```python
from build123d import *

# Parameters (mm, degrees)
SKETCH1_W                      = 40
SKETCH1_H                      = 45.36
BOSS_EXTRUDE1_DEPTH            = 14
SKETCH2_W                      = 29.2
SKETCH2_H                      = 38.5
CUT_EXTRUDE1_DEPTH             = 6.2
M2_5_CLEARANCE_HOLE1_OUTLINE_R = 1.45
M2_5_CLEARANCE_HOLE1_DEPTH     = 14
F_16_0MM_DOWEL_HOLE1_D         = 16
SKETCH11_R                     = 16
CUT_EXTRUDE2_DEPTH             = 63.076804041
CHAMFER1_SIZE                  = 6
FILLET1_R                      = 2


# Read off the part's stored shape, not the designer's step: M2.5 Clearance Hole1
with BuildPart() as part:
    # Sketch1 → Boss-Extrude1 (new body)
    with BuildSketch(Plane(origin=(0, 0, 0), x_dir=(1, 0, 0), z_dir=(0, 1, 0))):
        with Locations((20, 22.68)):
            Rectangle(SKETCH1_W, SKETCH1_H)
    extrude(amount=BOSS_EXTRUDE1_DEPTH)

    # Sketch2 → Cut-Extrude1 (cut)
    with BuildSketch(Plane(origin=(0, 14, 0), x_dir=(1, 0, 0), z_dir=(0, 1, 0))):
        with Locations((20, 26.11)):
            Rectangle(SKETCH2_W, SKETCH2_H)
    extrude(amount=-CUT_EXTRUDE1_DEPTH, mode=Mode.SUBTRACT)

    # M2.5 Clearance Hole1 outline → M2.5 Clearance Hole1 (cut)
    with BuildSketch(Plane(origin=(0, 0, 0), x_dir=(1, 0, 0), z_dir=(0, 1, 0))):
        with Locations((9, 4.2)):
            Circle(M2_5_CLEARANCE_HOLE1_OUTLINE_R)
        with Locations((31, 4.2)):
            Circle(M2_5_CLEARANCE_HOLE1_OUTLINE_R)
        with Locations((2.7, 34)):
            Circle(M2_5_CLEARANCE_HOLE1_OUTLINE_R)
        with Locations((2.7, 12)):
            Circle(M2_5_CLEARANCE_HOLE1_OUTLINE_R)
        with Locations((37.3, 12)):
            Circle(M2_5_CLEARANCE_HOLE1_OUTLINE_R)
        with Locations((37.3, 34)):
            Circle(M2_5_CLEARANCE_HOLE1_OUTLINE_R)
    extrude(amount=M2_5_CLEARANCE_HOLE1_DEPTH, mode=Mode.SUBTRACT)

    # Ø16.0mm Dowel Hole1 (through all)
    with Locations(Plane(origin=(0, 0, 0), x_dir=(-1, 0, 0), z_dir=(0, -1, 0))):
        with Locations((-20, 24)):
            Hole(F_16_0MM_DOWEL_HOLE1_D / 2)

    # Sketch11 → Cut-Extrude2 (cut, through all)
    with BuildSketch(Plane.XZ):
        with Locations((20, -52)):
            Circle(SKETCH11_R)
    extrude(amount=-CUT_EXTRUDE2_DEPTH, mode=Mode.SUBTRACT)

    # Chamfer1
    chamfer1_edges = [part.edges().sort_by_distance(p)[0] for p in [
        (0, 7, 0),
        (40, 7, 0),
    ]]
    chamfer(chamfer1_edges, length=CHAMFER1_SIZE)

    # Fillet1
    fillet1_edges = [part.edges().sort_by_distance(p)[0] for p in [
        (5.4, 10.9, -6.86),
        (34.6, 10.9, -6.86),
    ]]
    fillet(fillet1_edges, radius=FILLET1_R)


solid = part.part
```
Part model, mm, in its own coordinate system. A direction names the side the tool comes from. Give positions to 0.01 mm unless a question says otherwise; leave off trailing zeros. Write each loop counter-clockwise with the first axis right and the second up, starting at its lowest first coordinate (ties: lowest second). Pieces come first, ordered by that corner, then holes. Notation, with made-up numbers: M 26,-16.5 L 40,-16.5 A35 cw 40,18.5 Z; hole C 66.25,28 d10. An arc over 180 degrees is marked long. Use CSV: the item, a comma, the result in double quotes.
Item 1: Slice it at C-C on x = 20. Write the cut outline in (y, z).
Taken from the geometry:
outline,"M 0,-36 L 7.8,-36 L 7.8,-32 L 0,-32 Z; M 0,-16 L 7.8,-16 L 7.8,-6.86 L 14,-6.86 L 14,0 L 0,0 Z"
Item 2: Drill centre lines: probe 1 along X at (y, z) = (9.25, -12); probe 2 along X at (y, z) = (5.75, -12); probe 3 along X at (y, z) = (12.5, -22.5). Where is each one in solid material? Low to high.
Taken from the geometry:
probe 1,"x = 0 to 1.25, 4.15 to 5.4, 34.6 to 35.85, 38.75 to 40"
probe 2,"x = 0 to 1.25, 4.15 to 35.85, 38.75 to 40"
probe 3,"x = 0 to 5.4, 34.6 to 40"
Item 3: Slice it at B-B on z = -24. Write the cut outline in (x, y), plus the area to 3 significant figures.
Taken from the geometry:
outline,"M 0,0 L 12,0 L 12,7.8 L 5.4,7.8 L 5.4,14 L 0,14 Z; M 28,0 L 40,0 L 40,14 L 34.6,14 L 34.6,7.8 L 28,7.8 Z"
area,"254 mm²"
Item 4: Slice it at D-D on y = 12.75. Write the cut outline in (x, z).
Taken from the geometry:
outline,"M 0,-45.36 L 5.4,-45.36 L 5.4,-8.86 A2 cw 7.4,-6.86 L 32.6,-6.86 A2 cw 34.6,-8.86 L 34.6,-45.36 L 40,-45.36 L 40,-6 L 34,0 L 6,0 L 0,-6 Z; hole C 2.7,-34 d2.9; hole C 2.7,-12 d2.9; hole C 9,-4.2 d2.9; hole C 31,-4.2 d2.9; hole C 37.3,-34 d2.9; hole C 37.3,-12 d2.9"
Item 5: Pin check, flat tips, straight feed: P1, Ø1.9, axis at x = 21.5, y = 11.5, coming from the -Z side; P2, Ø1, axis at x = 17.5, z = -36, coming from the +Y side; P3, Ø1, axis at x = 27, y = 2.5, coming from the -Z side. Stop position of each tip, or through.
Taken from the geometry:
P1,"stops at z = -6.86"
P2,"stops at y = 7.8"
P3,"stops at z = -37.87"
Item 6: Pull direction X, two halves, no side cores. Call faces 1 (the face through (20, 14, -6)), 2 (the face through (3, 7, -3)), 3 (the face through (20, 11, -6.86)): +X half, -X half, draft (parallel to the pull), parting line (faces both ways), or undercut.
Taken from the geometry:
face 1,"draft"
face 2,"-X half"
face 3,"undercut"
Item 7: Which spindle directions (+Z, -Z, +X, -X, +Y, -Y) get a long thin tool onto all of the face, cutting with end or side? Do faces 4 (the face through (37, 7, -45.36)), 5 (the face through (5.4, 11, -27)). Say none if no direction does.
Taken from the geometry:
face 4,"-Z, +X, -X, +Y, -Y"
face 5,"-Z, +Y"
Item 8: Slice it at A-A on x = 2.7. Write the cut outline in (y, z), plus the area to 3 significant figures.
Taken from the geometry:
outline,"M 0,-45.36 L 14,-45.36 L 14,-35.45 L 0,-35.45 Z; M 0,-32.55 L 14,-32.55 L 14,-13.45 L 0,-13.45 Z; M 0,-10.55 L 14,-10.55 L 14,-3.3 L 0,-3.3 Z"
area,"508 mm²"
